Input: dimensioned drawing with shaded views. Units: mm. Origin: part minimum x, y, z. Round coordinates to 2 decimals unless told otherwise and drop trailing zeros. Loops run counter-clockwise (first coordinate to the right, second up) from the corner with the lowest first, then second, coordinate; pieces in that order, holes last. Notation, with made-up numbers: (4.25, -19) - (29.25, -19) arc R15 ccw to (29.25, -14) - close; hole circle Ø10 at (66.5, 1.25). An arc over 180 degrees is marked (long way). Use CSV: the item, a comma, the result in double quotes. Start each with the question number.
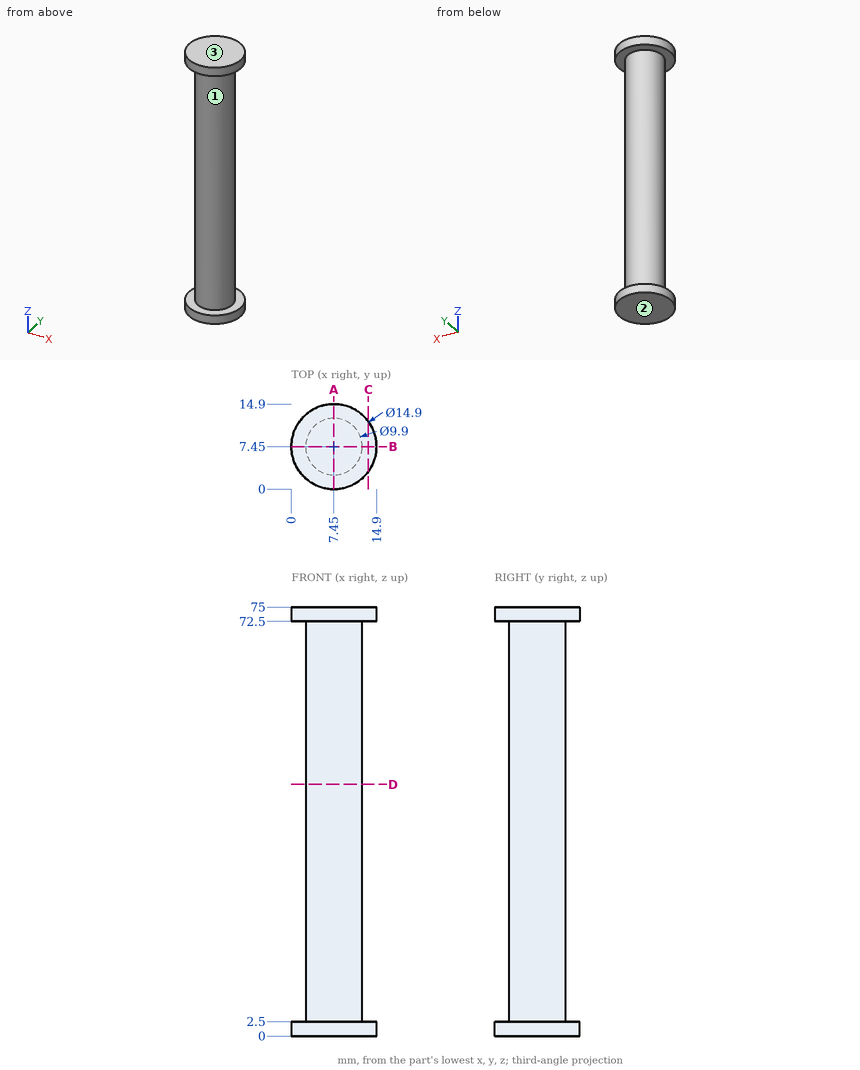
1. Mould query, pull axis Z, two halves, no side actions, for the marked faces 1, 2 and 3. Classes: +Z half, -Z half, draft (parallel to the pull), parting line (faces both ways), or undercut.
2. Section query D-D on z = 44. Return the cut outline in (x, y), and give its area (3 significant figures).
3. Section query C-C on x = 13.5. Return the cut outline in (y, z).
4. Line query: line 1 along Z through (x, y) = (1.75, 7.75); line 2 along X through (y, z) = (7.25, 24); line 3 along X through (y, z) = (4.75, 26.5). Output: solid intervals per line, ascending.
5. Section query A-A on x = 7.45. Return the cut outline in (y, z).
6. Contact query for flat-ended pins moving along their axis: P1, Ø1.5, axis at x = 12.5, y = 11.5, coming from the -Z side; P2, Ø4, axis at y = 5, z = 57, coming from the -X side; P3, Ø2, axis at y = 13, z = 60.5, coming from the -X side; P4, Ø5, axis at x = 5.5, z = 8, coming from the -Y side. Output: stop coordinate, or through.
Values:
1,face 1,"undercut"
1,face 2,"-Z half"
1,face 3,"+Z half"
2,outline,"circle Ø9.9 at (7.45, 7.45)"
2,area,"77.0 mm^2"
3,outline,"(3.1, 0) - (11.8, 0) - (11.8, 2.5) - (3.1, 2.5) - close; (3.1, 72.5) - (11.8, 72.5) - (11.8, 75) - (3.1, 75) - close"
4,line 1,"z = 0 to 2.5, 72.5 to 75"
4,line 2,"x = 2.5 to 12.4"
4,line 3,"x = 3.3 to 11.6"
5,outline,"(0, 0) - (14.9, 0) - (14.9, 2.5) - (12.4, 2.5) - (12.4, 72.5) - (14.9, 72.5) - (14.9, 75) - (0, 75) - (0, 72.5) - (2.5, 72.5) - (2.5, 2.5) - (0, 2.5) - close"
6,P1,"stops at z = 0"
6,P2,"stops at x = 2.52"
6,P3,"stops at x = 5.5"
6,P4,"stops at y = 2.5"
